Could you check a few things on this model? Use its own coordinates, in mm. A direction names the side the tool comes from. Give positions to 0.01 mm unless a question says otherwise; leave off trailing zeros. Order: outer loops, then holes, each group sorted by start corner. A loop starts at its lowest first (then second) coordinate and runs counter-clockwise, first axis right, second up.
from build123d import *

# Parameters (mm, degrees)
SKETCH1_R           = 10
BOSS_EXTRUDE1_DEPTH = 77.5
SKETCH2_W           = 12
SKETCH2_H           = 4
CUT_EXTRUDE1_DEPTH  = 3.2
SKETCH5_W           = 1.3
SKETCH5_H           = 0.5
SKETCH6_W           = 30
SKETCH6_H           = 20
CUT_EXTRUDE2_DEPTH  = 81.661329025


with BuildPart() as part:
    # Sketch1 → Boss-Extrude1 (new, symmetric)
    with BuildSketch(Plane(origin=(0, 0, 0), x_dir=(0, 0, -1), z_dir=(1, 0, 0))):
        Circle(SKETCH1_R)
    extrude(amount=BOSS_EXTRUDE1_DEPTH, both=True)

    # Sketch2 → Cut-Extrude1 (cut)
    with BuildSketch(Plane(origin=(0, 10, 0), x_dir=(1, 0, 0), z_dir=(0, 1, 0))):
        with Locations((-50.5, 0)):
            Rectangle(SKETCH2_W, SKETCH2_H)
        with Locations((-18.5, 0)):
            Rectangle(SKETCH2_W, SKETCH2_H)
        with Locations((66.5, 0)):
            Rectangle(SKETCH2_W, SKETCH2_H)
    extrude(amount=-CUT_EXTRUDE1_DEPTH, mode=Mode.SUBTRACT)

    # Sketch5 → Cut-Revolve2 (revolve, cut)
    with BuildSketch(Plane.XY, mode=Mode.PRIVATE) as cut_revolve2_sk:
        with Locations((-27.15, 9.75)):
            Rectangle(SKETCH5_W, SKETCH5_H)
        with Locations((-9.85, 9.75)):
            Rectangle(SKETCH5_W, SKETCH5_H)
        with Locations((75.15, 9.75)):
            Rectangle(SKETCH5_W, SKETCH5_H)
        with Locations((57.85, 9.75)):
            Rectangle(SKETCH5_W, SKETCH5_H)
        with Locations((35.85, 9.75)):
            Rectangle(SKETCH5_W, SKETCH5_H)
        with Locations((-68.5, 9.75)):
            Rectangle(SKETCH5_W, SKETCH5_H)
    revolve(cut_revolve2_sk.sketch.rotate(Axis((0, 0, 0), (-1, 0, 0)), 90), axis=Axis((0, 0, 0), (-1, 0, 0)), mode=Mode.SUBTRACT)

    # Sketch6 → Cut-Extrude2 (cut, through all)
    with BuildSketch(Plane(origin=(0, 10, 0), x_dir=(1, 0, 0), z_dir=(0, 1, 0))):
        with Locations((62.5, 0)):
            Rectangle(SKETCH6_W, SKETCH6_H)
    extrude(amount=-CUT_EXTRUDE2_DEPTH, mode=Mode.SUBTRACT)


solid = part.part
Item 1: We'd pull the mould along X, two halves only. Please class faces 4 (the flat face through (-19, 6.8, 0)), 5 (the flat face through (-77.5, 0, 0)), 6 (the cylindrical face through (-47.54, -9.76, 2.17)): +X half, -X half, draft (parallel to the pull), parting line (faces both ways), or undercut.
Findings:
face 4: undercut
face 5: -X half
face 6: draft
Item 2: For faces 1 (the flat face through (-27.8, 4, 9)), 2 (the flat face through (-44.5, 8, 0)), 3 (the cylindrical face through (13.31, -9.76, 2.17)), which set-ups out of +Z, -Z, +X, -X, +Y, -Y let a thin tool reach every point of the face, with its end or its side?
Findings:
face 1: none
face 2: +Y
face 3: +X, -X
Item 3: For pin 1 (12 mm diameter, centred on x = -48.5, z = -6.5, fed in from +Y); pin 2 (2 mm diameter, centred on x = -29.5, y = 6, fed in from +Z); pin 3 (1.5 mm diameter, centred on x = 33, z = 7.5, fed in from -Y), each with a flat end and sliding along its axis, tell me the tip position at first contact or that it passes through.
Findings:
pin 1: stops at y = 9.8
pin 2: stops at z = 8.66
pin 3: stops at y = -7.38
Item 4: Imagine slicing it at A-A on x = -54. List the corners of the cut face in (y, z) for me.
Findings:
outline: (6.8, -2) - (6.8, 2) - (9.8, 2) arc R10 ccw (long way) to (9.8, -2) - close
Item 5: Please list where these lines run through material, in increasing order: line 1 along Y through (x, z) = (21.5, -9); line 2 along Y through (x, z) = (-32, -4.25); line 3 along Z through (x, y) = (-24, -1.75).
Findings:
line 1: y = -4.36 to 4.36
line 2: y = -9.05 to 9.05
line 3: z = -9.85 to 9.85
